Design review of the part shown in the three views and the two pictorial views. Dimensions are in mm from the part's minimum x, y and z. Round coordinates to 2 decimals unless told otherwise and drop trailing zeros. Order: outer loops, then holes, each group sorted by start corner. A loop starts at its lowest first (then second) coordinate and runs counter-clockwise, first axis right, second up. Notation, with made-up numbers: M 37.5,65 L 44.5,65 A14 cw 44.5,72 Z; hole C -8.5,-10.75 d9. An arc over 180 degrees is marked long. Write each question's results on one line, items separated by ' | '. Start each with the question number.
Item 1: Wall thickness on line 1 (Z direction, x = 13.25, y = 35.5); line 2 (Z direction, x = 1.25, y = 45); line 3 (Z direction, x = 14, y = 57.5): over which ranges is each line inside the solid? List them lowest first. Write a range as [from, to].
Item 2: The part is to be moulded in two halves that separate along X. For the marked faces 1, 2 and 3, say which applies: +X half, -X half, draft (parallel to the pull), parting line (faces both ways), or undercut.
Item 3: Clearance check with flat-ended pins moving along their axes: pin 1 (1.5 mm diameter, centred on x = 16.5, y = 2, fed in from +Z); pin 2 (5.5 mm diameter, centred on y = 7.5, z = 22, fed in from +X); pin 3 (2.5 mm diameter, centred on x = 12, z = 57, fed in from -Y); pin 4 (12 mm diameter, centred on y = 33.5, z = 16.5, fed in from -X). State where each tip first meets the part, or that it passes through.
Item 4: Take a section at A-A, the plane z = 29. Write out the cut boundary in (x, y).
Item 5: Take a section at D-D, the plane z = 22. Write out the cut boundary in (x, y) (1 decimal), plus the area to 3 significant figures.
Item 6: Take a section at B-B, the plane y = 9.5. Write out the cut boundary in (x, z).
Item 7: Take a section at C-C, the plane x = 11.5. Write out the cut boundary in (y, z), plus the area to 3 significant figures.
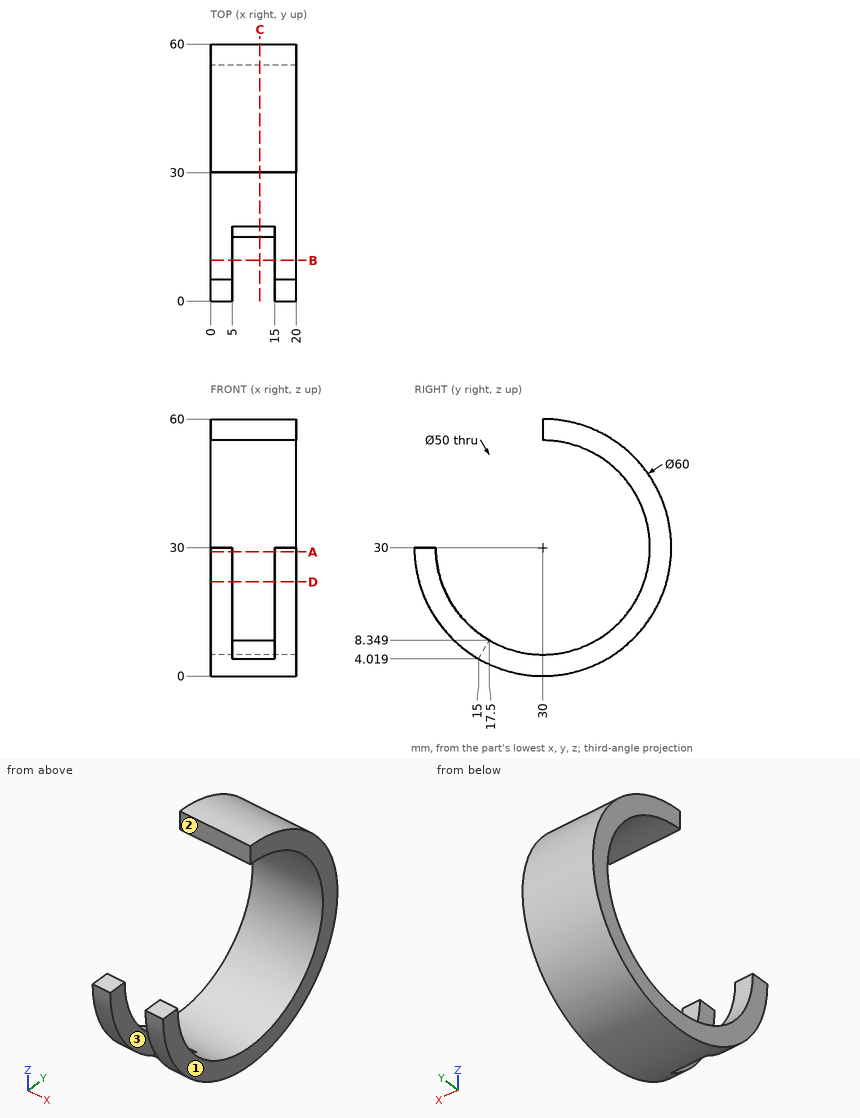
Results list:
1) line 1: [0.51, 5.61], [54.39, 59.49] | line 2: [4.02, 10], [50, 55.98] | line 3: [18.01, 41.99]
2) face 1: +X half | face 2: draft | face 3: undercut
3) pin 1: z = 30 | pin 2: x = 20 | pin 3: y = 30 | pin 4: through
4) outline: M 0,0.02 L 5,0.02 L 5,5.02 L 0,5.02 Z; M 0,54.98 L 20,54.98 L 20,59.98 L 0,59.98 Z; M 15,0.02 L 20,0.02 L 20,5.02 L 15,5.02 Z
5) outline: M 0,1.1 L 5,1.1 L 5,6.3 L 0,6.3 Z; M 0,53.7 L 20,53.7 L 20,58.9 L 0,58.9 Z; M 15,1.1 L 20,1.1 L 20,6.3 L 15,6.3 Z | area: 157 mm²
6) outline: M 0,8.1 L 5,8.1 L 5,15.69 L 0,15.69 Z; M 15,8.1 L 20,8.1 L 20,15.69 L 15,15.69 Z
7) outline: M 15,4.02 A30 ccw long 30,60 L 30,55 A25 cw long 17.5,8.35 Z | area: 504 mm²
